```python
from build123d import *

# Parameters (mm, degrees)
F0_W     = 22
F0_H     = 17
F1_DEPTH = 3
F2_W     = 22
F2_H     = 2
F3_DEPTH = 10
F4_W     = 22
F4_H     = 1
F7_R     = 1


with BuildPart() as f1:
    # F0 (on Top) → F1 (new body)
    with BuildSketch(Plane.XY):
        Rectangle(F0_W, F0_H)
    extrude(amount=F1_DEPTH)

    # F2 (on face) → F3 (join)
    with BuildSketch(Plane.XY.offset(3)):
        with Locations((0, 2.5)):
            Rectangle(F2_W, F2_H)
        with Locations((0, -2.5)):
            Rectangle(F2_W, F2_H)
    extrude(amount=F3_DEPTH)

    # F4 (on face) → F5 (revolve)
    with BuildSketch(Plane.XZ.offset(-1.5)):
        with Locations((0, 12.5)):
            Rectangle(F4_W, F4_H)
    revolve(axis=Axis((0, 1.5, 12), (-1, 0, 0)))

    # F6: F1 across plane


with BuildPart() as f1_1:
    add(f1.part)
    add(f1.part.mirror(Plane.XZ))

    # F7
    f7_edges = [f1_1.edges().sort_by_distance(p)[0] for p in [
        (0, -3.5, 3),
        (0, -3.5, 13),
        (11, 3.5, 8),
        (11, -6, 3),
        (0, -8.5, 3),
        (-11, -6, 3),
        (0, 3.5, 13),
        (0, 3.5, 3),
        (-11, 6, 3),
        (11, 6, 3),
        (0, 8.5, 3),
        (-11, 3.5, 8),
        (-11, -3.5, 8),
        (11, -3.5, 8),
    ]]
    fillet(f7_edges, radius=F7_R)


solid = f1_1.part
```
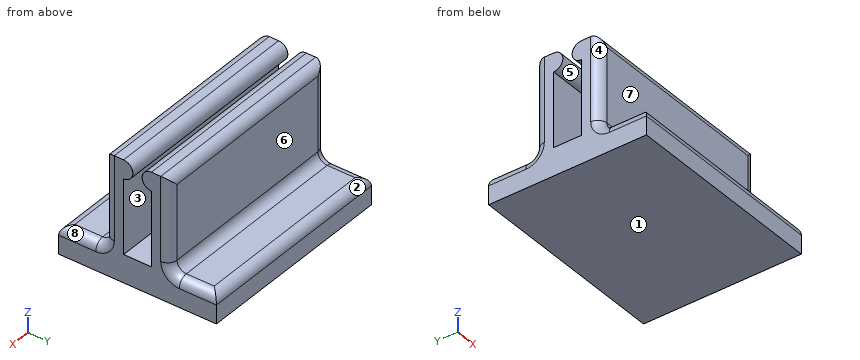
The model under review builds one solid part; all positions refer to its coordinate system, in mm. Face numbers are marked on the shaded views. A direction names the side the tool comes from. Round coordinates to 2 decimals unless told otherwise and drop trailing zeros. Write each loop counter-clockwise with the first axis right and the second up, starting at its lowest first coordinate (ties: lowest second). Pieces come first, ordered by that corner, then holes. Notation, with made-up numbers: (-28.5, 22.5) - (-16.5, 22.5) arc R26 ccw to (-16.5, 50.5) - close; hole circle Ø7 at (60, -14.75). An arc over 180 degrees is marked (long way). One line per question, with ' | ' between items.
Item 1: For P1, Ø4, axis at x = -2.5, z = 6, coming from the -Y side; P2, Ø3, axis at x = -4.5, z = 8.5, coming from the +Y side; P3, Ø2.5, axis at x = -4, y = 6.5, coming from the +Z side; P4, Ø4, axis at x = -4.5, z = 4, coming from the -Y side, all flat-tipped, find the tip position at first contact; note any pin that passes through.
Resolved:
P1: stops at y = -3.5 | P2: stops at y = 3.5 | P3: stops at z = 3 | P4: stops at y = -8.5
Item 2: Add section C-C, the plane x = 8.25. Give the boundary of the cut face in (y, z).
Resolved:
outline: (-8.5, 0) - (8.5, 0) - (8.5, 2) arc R1 ccw to (7.5, 3) - (4.5, 3) arc R1 cw to (3.5, 4) - (3.5, 12) arc R1 ccw to (2.5, 13) - (1.5, 13) arc R1 ccw to (1.5, 11) - (1.5, 3) - (-1.5, 3) - (-1.5, 11) arc R1 ccw to (-1.5, 13) - (-2.5, 13) arc R1 ccw to (-3.5, 12) - (-3.5, 4) arc R1 cw to (-4.5, 3) - (-7.5, 3) arc R1 ccw to (-8.5, 2) - close
Item 3: The part is to be moulded in two halves that separate along Z. For the marked faces 1, 2 and 3, say which applies: pulls with the +Z half, pulls with the -Z half, needs draft (parallel to the pull), parting line crosses it, or undercut.
Resolved:
face 1: pulls with the -Z half | face 2: pulls with the +Z half | face 3: undercut
Item 4: To check wall thickness, follow probe 1 along Y at (x, z) = (-7, 5.5); probe 2 along Z at (x, y) = (-2.25, -5.75); probe 3 along Z at (x, y) = (-1.25, 0.75). State the ranges of each line that lie inside material, in increasing order.
Resolved:
probe 1: y = -3.5 to -1.5, 1.5 to 3.5 | probe 2: z = 0 to 3 | probe 3: z = 0 to 3, 11.34 to 12.66
Item 5: Add section A-A, the plane z = 6.5. Give the boundary of the cut face in (x, y), then the cut area to 3 significant figures.
Resolved:
outline: (-11, -2.5) arc R1 ccw to (-10, -3.5) - (10, -3.5) arc R1 ccw to (11, -2.5) - (11, -1.5) - (-11, -1.5) - close; (-11, 1.5) - (11, 1.5) - (11, 2.5) arc R1 ccw to (10, 3.5) - (-10, 3.5) arc R1 ccw to (-11, 2.5) - close | area: 87.1 mm2
Item 6: Add section B-B, the plane y = -1. Give the boundary of the cut face in (x, z), then the cut area to 3 significant figures.
Resolved:
outline: (-11, 0) - (11, 0) - (11, 3) - (-11, 3) - close; (-11, 11.13) - (11, 11.13) - (11, 12.87) - (-11, 12.87) - close | area: 104 mm2
Item 7: For the marked faces 4, 5, 6, 7 and 8, list the 3-axis set-ups (+Z, -Z, +X, -X, +Y, -Y) from which the entire face can be reached by the end or side of a thin tool; tool diameter is ignored.
Resolved:
face 4: +Z, -X, -Y | face 5: +X, -X | face 6: +Z, +X, -X, +Y | face 7: +Z, +X, -X, -Y | face 8: +Z, +X, -Y
Item 8: Add section D-D, the plane y = 6. Give the boundary of the cut face in (x, z), then the cut area to 3 significant figures.
Resolved:
outline: (-11, 0) - (11, 0) - (11, 2) arc R1 ccw to (10, 3) - (-10, 3) arc R1 ccw to (-11, 2) - close | area: 65.6 mm2
